Could you check a few things on this model? Use its own coordinates, in mm. A direction names the side the tool comes from. Give positions to 0.01 mm unless a question says otherwise; leave off trailing zeros. Order: outer loops, then holes, each group sorted by start corner. A loop starts at its lowest first (then second) coordinate and runs counter-clockwise, first axis right, second up.
from build123d import *

# Parameters (mm, degrees)
SKETCH2_W           = 20.5
SKETCH2_H           = 41
BOSS_EXTRUDE1_DEPTH = 42.5
BOSS_EXTRUDE2_START = 33.4
SKETCH2_3_W         = 20.5
SKETCH2_3_H         = 41
BOSS_EXTRUDE2_DEPTH = 4.1


with BuildPart() as part:
    # Sketch2 → Boss-Extrude1 (new body)
    with BuildSketch(Plane(origin=(0, 0, 0), x_dir=(1, 0, 0), z_dir=(0, 1, 0))):
        Rectangle(SKETCH2_W, SKETCH2_H)
    extrude(amount=BOSS_EXTRUDE1_DEPTH)

    # Sketch2_3 → Boss-Extrude2 (add)
    with BuildSketch(Plane(origin=(0, 0, 0), x_dir=(1, 0, 0), z_dir=(0, 1, 0)).offset(BOSS_EXTRUDE2_START)):
        with BuildLine():
            Line((-10.25, 28), (-10.25, 20.5))
            Line((-10.25, 20.5), (10.25, 20.5))
            Line((10.25, 20.5), (10.25, 28))
            Line((10.25, 28), (6.715, 28))
            Line((6.715, 28), (6.715, 26.825661404))
            ThreePointArc((6.715, 26.825661404), (5.55, 23.2), (4.385, 26.825661404))
            Line((4.385, 26.825661404), (4.385, 28))
            Line((4.385, 28), (-4.385, 28))
            Line((-4.385, 28), (-4.385, 26.825661404))
            ThreePointArc((-4.385, 26.825661404), (-5.55, 23.2), (-6.715, 26.825661404))
            Line((-6.715, 26.825661404), (-6.715, 28))
            Line((-6.715, 28), (-10.25, 28))
        make_face()
        Rectangle(SKETCH2_3_W, SKETCH2_3_H)
        with BuildLine():
            Line((10.25, -20.5), (-10.25, -20.5))
            Line((-10.25, -20.5), (-10.25, -28))
            Line((-10.25, -28), (-6.715, -28))
            Line((-6.715, -28), (-6.715, -26.825661404))
            ThreePointArc((-6.715, -26.825661404), (-5.55, -23.2), (-4.385, -26.825661404))
            Line((-4.385, -26.825661404), (-4.385, -28))
            Line((-4.385, -28), (4.385, -28))
            Line((4.385, -28), (4.385, -26.825661404))
            ThreePointArc((4.385, -26.825661404), (5.55, -23.2), (6.715, -26.825661404))
            Line((6.715, -26.825661404), (6.715, -28))
            Line((6.715, -28), (10.25, -28))
            Line((10.25, -28), (10.25, -20.5))
        make_face()
    extrude(amount=BOSS_EXTRUDE2_DEPTH)


solid = part.part
Item 1: Imagine slicing it at D-D on y = 4. List the corners of the cut face in (x, z) for me, then the cut area to 4 significant figures.
Findings:
outline: (-10.25, -20.5) - (10.25, -20.5) - (10.25, 20.5) - (-10.25, 20.5) - close
area: 840.5 mm2
Item 2: Please list where these lines run through material, in increasing order: line 1 along X through (y, z) = (34, -25); line 2 along Z through (x, y) = (-5.75, 39.5); line 3 along Y through (x, z) = (-1.25, -24.5).
Findings:
line 1: x = -10.25 to -7.54, -3.56 to 3.56, 7.54 to 10.25
line 2: z = -20.5 to 20.5
line 3: y = 33.4 to 37.5
Item 3: For pin 1 (12 mm diameter, centred on x = 4.5, y = 18, fed in from -Z); pin 2 (4.5 mm diameter, centred on x = -5.55, z = 25.2, fed in from -Y); pin 3 (6 mm diameter, centred on x = 1, y = 9, fed in from +Z), each with a flat end and sliding along its axis, tell me the tip position at first contact or that it passes through.
Findings:
pin 1: stops at z = -20.5
pin 2: stops at y = 33.4
pin 3: stops at z = 20.5
Item 4: Imagine slicing it at C-C on x = 8.5. List the corners of the cut face in (y, z) for me, then the cut area to 3 significant figures.
Findings:
outline: (0, -20.5) - (33.4, -20.5) - (33.4, -28) - (37.5, -28) - (37.5, -20.5) - (42.5, -20.5) - (42.5, 20.5) - (37.5, 20.5) - (37.5, 28) - (33.4, 28) - (33.4, 20.5) - (0, 20.5) - close
area: 1,800 mm2
Item 5: For faces 1 (the flat face through (-4.385, 35, -27)), 2 (the flat face through (4.385, 35, 27)), 3 (the flat face through (0, 40, 20.5)), which set-ups out of +Z, -Z, +X, -X, +Y, -Y let a thin tool reach every point of the face, with its end or its side?
Findings:
face 1: -Z, +Y, -Y
face 2: +Z, +Y, -Y
face 3: +Z, +X, -X, +Y
Item 6: Imagine slicing it at B-B on x = 5.55. List the corners of the cut face in (y, z) for me, then the cut area to 3 significant figures.
Findings:
outline: (0, -20.5) - (33.4, -20.5) - (33.4, -23.2) - (37.5, -23.2) - (37.5, -20.5) - (42.5, -20.5) - (42.5, 20.5) - (37.5, 20.5) - (37.5, 23.2) - (33.4, 23.2) - (33.4, 20.5) - (0, 20.5) - close
area: 1,760 mm2
Item 7: We'd pull the mould along Z, two halves only. Please class faces 4 (the flat face through (8, 35, 28)), 5 (the cylindrical face through (-5.5, 35.4, -23.2)), 6 (the flat face through (0, 35, -28)), 7 (the cylindrical face through (5.5, 35.4, 23.2)): +Z half, -Z half, draft (parallel to the pull), parting line (faces both ways), or undercut.
Findings:
face 4: +Z half
face 5: undercut
face 6: -Z half
face 7: undercut
Item 8: Imagine slicing it at A-A on z = 25.2. List the corners of the cut face in (x, y) for me, then the cut area to 4 significant figures.
Findings:
outline: (-10.25, 33.4) - (-7.55, 33.4) - (-7.55, 37.5) - (-10.25, 37.5) - close; (-3.55, 33.4) - (3.55, 33.4) - (3.55, 37.5) - (-3.55, 37.5) - close; (7.55, 33.4) - (10.25, 33.4) - (10.25, 37.5) - (7.55, 37.5) - close
area: 51.25 mm2
